from build123d import *

# Parameters (mm, degrees)
F0_W     = 374.219984
F0_H     = 260
F1_DEPTH = 3


with BuildPart() as f1:
    # F0 (on Top) → F1 (new body)
    with BuildSketch(Plane.XY):
        with Locations((162.909992, -105.8)):
            Rectangle(F0_W, F0_H)
        with BuildLine():
            ThreePointArc((14.186787, -200.612439), (-12.519984, -206.7), (7.360575, -187.856609))
            ThreePointArc((7.360575, -187.856609), (19.132652, -189.761268), (14.186787, -200.612439))
        make_face(mode=Mode.SUBTRACT)
        with BuildLine():
            ThreePointArc((54.186787, -200.612439), (27.480016, -206.7), (47.360575, -187.856609))
            ThreePointArc((47.360575, -187.856609), (59.132652, -189.761268), (54.186787, -200.612439))
        make_face(mode=Mode.SUBTRACT)
        with BuildLine():
            ThreePointArc((94.186787, -200.612439), (67.480016, -206.7), (87.360575, -187.856609))
            ThreePointArc((87.360575, -187.856609), (99.132652, -189.761268), (94.186787, -200.612439))
        make_face(mode=Mode.SUBTRACT)
        with BuildLine():
            ThreePointArc((134.186787, -200.612439), (107.480016, -206.7), (127.360575, -187.856609))
            ThreePointArc((127.360575, -187.856609), (139.132652, -189.761268), (134.186787, -200.612439))
        make_face(mode=Mode.SUBTRACT)
        with BuildLine():
            ThreePointArc((174.186787, -200.612439), (147.480016, -206.7), (167.360575, -187.856609))
            ThreePointArc((167.360575, -187.856609), (179.132652, -189.761268), (174.186787, -200.612439))
        make_face(mode=Mode.SUBTRACT)
        with BuildLine():
            ThreePointArc((214.186787, -200.612439), (187.480016, -206.7), (207.360575, -187.856609))
            ThreePointArc((207.360575, -187.856609), (219.132652, -189.761268), (214.186787, -200.612439))
        make_face(mode=Mode.SUBTRACT)
        with BuildLine():
            ThreePointArc((14.186787, -150.612439), (-12.519984, -156.7), (7.360575, -137.856609))
            ThreePointArc((7.360575, -137.856609), (19.132652, -139.761268), (14.186787, -150.612439))
        make_face(mode=Mode.SUBTRACT)
        with BuildLine():
            ThreePointArc((54.186787, -150.612439), (27.480016, -156.7), (47.360575, -137.856609))
            ThreePointArc((47.360575, -137.856609), (59.132652, -139.761268), (54.186787, -150.612439))
        make_face(mode=Mode.SUBTRACT)
        with BuildLine():
            ThreePointArc((94.186787, -150.612439), (67.480016, -156.7), (87.360575, -137.856609))
            ThreePointArc((87.360575, -137.856609), (99.132652, -139.761268), (94.186787, -150.612439))
        make_face(mode=Mode.SUBTRACT)
        with BuildLine():
            ThreePointArc((134.186787, -150.612439), (107.480016, -156.7), (127.360575, -137.856609))
            ThreePointArc((127.360575, -137.856609), (139.132652, -139.761268), (134.186787, -150.612439))
        make_face(mode=Mode.SUBTRACT)
        with BuildLine():
            ThreePointArc((174.186787, -150.612439), (147.480016, -156.7), (167.360575, -137.856609))
            ThreePointArc((167.360575, -137.856609), (179.132652, -139.761268), (174.186787, -150.612439))
        make_face(mode=Mode.SUBTRACT)
        with BuildLine():
            ThreePointArc((214.186787, -150.612439), (187.480016, -156.7), (207.360575, -137.856609))
            ThreePointArc((207.360575, -137.856609), (219.132652, -139.761268), (214.186787, -150.612439))
        make_face(mode=Mode.SUBTRACT)
        with BuildLine():
            ThreePointArc((254.186787, -200.612439), (227.480016, -206.7), (247.360575, -187.856609))
            ThreePointArc((247.360575, -187.856609), (259.132652, -189.761268), (254.186787, -200.612439))
        make_face(mode=Mode.SUBTRACT)
        with BuildLine():
            ThreePointArc((294.186787, -200.612439), (267.480016, -206.7), (287.360575, -187.856609))
            ThreePointArc((287.360575, -187.856609), (299.132652, -189.761268), (294.186787, -200.612439))
        make_face(mode=Mode.SUBTRACT)
        with BuildLine():
            ThreePointArc((334.186787, -200.612439), (307.480016, -206.7), (327.360575, -187.856609))
            ThreePointArc((327.360575, -187.856609), (339.132652, -189.761268), (334.186787, -200.612439))
        make_face(mode=Mode.SUBTRACT)
        with BuildLine():
            ThreePointArc((254.186787, -150.612439), (227.480016, -156.7), (247.360575, -137.856609))
            ThreePointArc((247.360575, -137.856609), (259.132652, -139.761268), (254.186787, -150.612439))
        make_face(mode=Mode.SUBTRACT)
        with BuildLine():
            ThreePointArc((294.186787, -150.612439), (267.480016, -156.7), (287.360575, -137.856609))
            ThreePointArc((287.360575, -137.856609), (299.132652, -139.761268), (294.186787, -150.612439))
        make_face(mode=Mode.SUBTRACT)
        with BuildLine():
            ThreePointArc((334.186787, -150.612439), (307.480016, -156.7), (327.360575, -137.856609))
            ThreePointArc((327.360575, -137.856609), (339.132652, -139.761268), (334.186787, -150.612439))
        make_face(mode=Mode.SUBTRACT)
        with BuildLine():
            ThreePointArc((14.186787, -100.612439), (-12.519984, -106.7), (7.360575, -87.856609))
            ThreePointArc((7.360575, -87.856609), (19.132652, -89.761268), (14.186787, -100.612439))
        make_face(mode=Mode.SUBTRACT)
        with BuildLine():
            ThreePointArc((54.186787, -100.612439), (27.480016, -106.7), (47.360575, -87.856609))
            ThreePointArc((47.360575, -87.856609), (59.132652, -89.761268), (54.186787, -100.612439))
        make_face(mode=Mode.SUBTRACT)
        with BuildLine():
            ThreePointArc((94.186787, -100.612439), (67.480016, -106.7), (87.360575, -87.856609))
            ThreePointArc((87.360575, -87.856609), (99.132652, -89.761268), (94.186787, -100.612439))
        make_face(mode=Mode.SUBTRACT)
        with BuildLine():
            ThreePointArc((14.186787, -50.612439), (-12.519984, -56.7), (7.360575, -37.856609))
            ThreePointArc((7.360575, -37.856609), (19.132652, -39.761268), (14.186787, -50.612439))
        make_face(mode=Mode.SUBTRACT)
        with BuildLine():
            ThreePointArc((54.186787, -50.612439), (27.480016, -56.7), (47.360575, -37.856609))
            ThreePointArc((47.360575, -37.856609), (59.132652, -39.761268), (54.186787, -50.612439))
        make_face(mode=Mode.SUBTRACT)
        with BuildLine():
            ThreePointArc((94.186787, -50.612439), (67.480016, -56.7), (87.360575, -37.856609))
            ThreePointArc((87.360575, -37.856609), (99.132652, -39.761268), (94.186787, -50.612439))
        make_face(mode=Mode.SUBTRACT)
        with BuildLine():
            ThreePointArc((134.186787, -100.612439), (107.480016, -106.7), (127.360575, -87.856609))
            ThreePointArc((127.360575, -87.856609), (139.132652, -89.761268), (134.186787, -100.612439))
        make_face(mode=Mode.SUBTRACT)
        with BuildLine():
            ThreePointArc((174.186787, -100.612439), (147.480016, -106.7), (167.360575, -87.856609))
            ThreePointArc((167.360575, -87.856609), (179.132652, -89.761268), (174.186787, -100.612439))
        make_face(mode=Mode.SUBTRACT)
        with BuildLine():
            ThreePointArc((214.186787, -100.612439), (187.480016, -106.7), (207.360575, -87.856609))
            ThreePointArc((207.360575, -87.856609), (219.132652, -89.761268), (214.186787, -100.612439))
        make_face(mode=Mode.SUBTRACT)
        with BuildLine():
            ThreePointArc((134.186787, -50.612439), (107.480016, -56.7), (127.360575, -37.856609))
            ThreePointArc((127.360575, -37.856609), (139.132652, -39.761268), (134.186787, -50.612439))
        make_face(mode=Mode.SUBTRACT)
        with BuildLine():
            ThreePointArc((174.186787, -50.612439), (147.480016, -56.7), (167.360575, -37.856609))
            ThreePointArc((167.360575, -37.856609), (179.132652, -39.761268), (174.186787, -50.612439))
        make_face(mode=Mode.SUBTRACT)
        with BuildLine():
            ThreePointArc((214.186787, -50.612439), (187.480016, -56.7), (207.360575, -37.856609))
            ThreePointArc((207.360575, -37.856609), (219.132652, -39.761268), (214.186787, -50.612439))
        make_face(mode=Mode.SUBTRACT)
        with BuildLine():
            ThreePointArc((14.186787, -0.612439), (-12.519984, -6.7), (7.360575, 12.143391))
            ThreePointArc((7.360575, 12.143391), (19.132652, 10.238732), (14.186787, -0.612439))
        make_face(mode=Mode.SUBTRACT)
        with BuildLine():
            ThreePointArc((54.186787, -0.612439), (27.480016, -6.7), (47.360575, 12.143391))
            ThreePointArc((47.360575, 12.143391), (59.132652, 10.238732), (54.186787, -0.612439))
        make_face(mode=Mode.SUBTRACT)
        with BuildLine():
            ThreePointArc((94.186787, -0.612439), (67.480016, -6.7), (87.360575, 12.143391))
            ThreePointArc((87.360575, 12.143391), (99.132652, 10.238732), (94.186787, -0.612439))
        make_face(mode=Mode.SUBTRACT)
        with BuildLine():
            ThreePointArc((134.186787, -0.612439), (107.480016, -6.7), (127.360575, 12.143391))
            ThreePointArc((127.360575, 12.143391), (139.132652, 10.238732), (134.186787, -0.612439))
        make_face(mode=Mode.SUBTRACT)
        with BuildLine():
            ThreePointArc((174.186787, -0.612439), (147.480016, -6.7), (167.360575, 12.143391))
            ThreePointArc((167.360575, 12.143391), (179.132652, 10.238732), (174.186787, -0.612439))
        make_face(mode=Mode.SUBTRACT)
        with BuildLine():
            ThreePointArc((214.186787, -0.612439), (187.480016, -6.7), (207.360575, 12.143391))
            ThreePointArc((207.360575, 12.143391), (219.132652, 10.238732), (214.186787, -0.612439))
        make_face(mode=Mode.SUBTRACT)
        with BuildLine():
            ThreePointArc((254.186787, -100.612439), (227.480016, -106.7), (247.360575, -87.856609))
            ThreePointArc((247.360575, -87.856609), (259.132652, -89.761268), (254.186787, -100.612439))
        make_face(mode=Mode.SUBTRACT)
        with BuildLine():
            ThreePointArc((294.186787, -100.612439), (267.480016, -106.7), (287.360575, -87.856609))
            ThreePointArc((287.360575, -87.856609), (299.132652, -89.761268), (294.186787, -100.612439))
        make_face(mode=Mode.SUBTRACT)
        with BuildLine():
            ThreePointArc((334.186787, -100.612439), (307.480016, -106.7), (327.360575, -87.856609))
            ThreePointArc((327.360575, -87.856609), (339.132652, -89.761268), (334.186787, -100.612439))
        make_face(mode=Mode.SUBTRACT)
        with BuildLine():
            ThreePointArc((254.186787, -50.612439), (227.480016, -56.7), (247.360575, -37.856609))
            ThreePointArc((247.360575, -37.856609), (259.132652, -39.761268), (254.186787, -50.612439))
        make_face(mode=Mode.SUBTRACT)
        with BuildLine():
            ThreePointArc((294.186787, -50.612439), (267.480016, -56.7), (287.360575, -37.856609))
            ThreePointArc((287.360575, -37.856609), (299.132652, -39.761268), (294.186787, -50.612439))
        make_face(mode=Mode.SUBTRACT)
        with BuildLine():
            ThreePointArc((334.186787, -50.612439), (307.480016, -56.7), (327.360575, -37.856609))
            ThreePointArc((327.360575, -37.856609), (339.132652, -39.761268), (334.186787, -50.612439))
        make_face(mode=Mode.SUBTRACT)
        with BuildLine():
            ThreePointArc((254.186787, -0.612439), (227.480016, -6.7), (247.360575, 12.143391))
            ThreePointArc((247.360575, 12.143391), (259.132652, 10.238732), (254.186787, -0.612439))
        make_face(mode=Mode.SUBTRACT)
        with BuildLine():
            ThreePointArc((294.186787, -0.612439), (267.480016, -6.7), (287.360575, 12.143391))
            ThreePointArc((287.360575, 12.143391), (299.132652, 10.238732), (294.186787, -0.612439))
        make_face(mode=Mode.SUBTRACT)
        with BuildLine():
            ThreePointArc((334.186787, -0.612439), (307.480016, -6.7), (327.360575, 12.143391))
            ThreePointArc((327.360575, 12.143391), (339.132652, 10.238732), (334.186787, -0.612439))
        make_face(mode=Mode.SUBTRACT)
    extrude(amount=F1_DEPTH)


solid = f1.part
Geometry: final body of the model. Coordinates: model frame, mm. Give positions to 0.01 mm unless a question says otherwise; leave off trailing zeros. Write each loop counter-clockwise with the first axis right and the second up, starting at its lowest first coordinate (ties: lowest second). Pieces come first, ordered by that corner, then holes.
(1) Cut plane C-C, the plane y = -143.3. Give the number of separate pieces and of enclosed holes in the cut face, then the cut area to 3 significant figures.
(2) Ray query, line 1 (Y direction, x = 120, z = 1.55); line 2 (Y direction, x = 137, z = 1.8). Return the intervals inside material, ascending.
(3) First-contact query: P1, Ø17, axis at x = 160, y = 0, coming from the -Z side. Flat tip, straight axial feed; report the tip coordinate or a pass-through.
(4) Cut plane B-B, the plane x = 322. Return loops of the section in (y, z).
(5) Cut plane A-A, the plane x = 200. Return loops of the section in (y, z), then the cut area to 3 significant figures.
Values follow:
1. separate pieces: 10
1. enclosed holes: 0
1. area: 244 mm2
2. line 1: y = -235.8 to -214.2, -185.8 to -164.2, -135.8 to -114.2, -85.8 to -64.2, -35.8 to -14.2, 14.2 to 24.2
2. line 2: y = -235.8 to -199.31, -187.29 to -149.31, -137.29 to -99.31, -87.29 to -49.31, -37.29 to 0.69, 12.71 to 24.2
3. P1: passes through
4. outline: (-235.8, 0) - (-214.06, 0) - (-214.06, 3) - (-235.8, 3) - close; (-185.94, 0) - (-164.06, 0) - (-164.06, 3) - (-185.94, 3) - close; (-135.94, 0) - (-114.06, 0) - (-114.06, 3) - (-135.94, 3) - close; (-85.94, 0) - (-64.06, 0) - (-64.06, 3) - (-85.94, 3) - close; (-35.94, 0) - (-14.06, 0) - (-14.06, 3) - (-35.94, 3) - close; (14.06, 0) - (24.2, 0) - (24.2, 3) - (14.06, 3) - close
5. outline: (-235.8, 0) - (-214.2, 0) - (-214.2, 3) - (-235.8, 3) - close; (-185.8, 0) - (-164.2, 0) - (-164.2, 3) - (-185.8, 3) - close; (-135.8, 0) - (-114.2, 0) - (-114.2, 3) - (-135.8, 3) - close; (-85.8, 0) - (-64.2, 0) - (-64.2, 3) - (-85.8, 3) - close; (-35.8, 0) - (-14.2, 0) - (-14.2, 3) - (-35.8, 3) - close; (14.2, 0) - (24.2, 0) - (24.2, 3) - (14.2, 3) - close
5. area: 354 mm2
